from build123d import *

# Parameters (mm, degrees)
F4_R     = 2.9
F5_DEPTH = 75.0134427933
F6_SIZE  = 1.5
F7_COUNT = 3


with BuildPart() as f1:
    # F0 (on Front) → F1 (revolve)
    with BuildSketch(Plane.XZ):
        Polygon((-9.15, 1), (-9.15, 25), (-14, 25), (-25, 14.5), (-25, 10.5), (-14, 0), (-10.15, 0), (-10.15, 1), align=None)
    revolve(axis=Axis((0, 0, 12.5), (0, 0, -1)))

    # F2 (on Front) → F3 (revolve)
    with BuildSketch(Plane.XZ):
        Polygon((-35.94647469, -20.5244732297), (-15.2322022896, 1.1761930946), (-10.7806652787, 5.8397080583), (-15.0484629892, 9.9135149637), (-19.5, 5.25), (-40.2142724005, -16.4506663243), align=None)
    revolve(axis=Axis((-29.8571362002, 0, -5.6003331622), (0.6904757467, 0, 0.7233555441)))

    # F4 (on face) → F5 (cut, through all)
    with BuildSketch(Plane(origin=(-27.3888669951, 0, -28.6930987567), x_dir=(0.7233555441, 0, -0.6904757467), z_dir=(-0.6904757467, 0, -0.7233555441))):
        with Locations((-17.7304307809, 0)):
            Circle(F4_R)
    extrude(amount=-F5_DEPTH, mode=Mode.SUBTRACT)

    # F6
    f6_edges = [f1.edges().sort_by_distance(p)[0] for p in [
        (-44.48207, 0, -12.376859),
    ]]
    chamfer(f6_edges, length=F6_SIZE)

    # F7: F1 ×3 about axis
    f7_axis = Axis((0, 0, 14.5), (0, 0, -1))


with BuildPart() as f1_1:
    add(f1.part)
    for i in range(1, F7_COUNT):
        add(f1.part.rotate(f7_axis, i * 360 / F7_COUNT))


solid = f1_1.part
The model under review builds one solid part; all positions refer to its coordinate system, in mm. A direction names the side the tool comes from. Round coordinates to 2 decimals unless told otherwise and drop trailing zeros. Order: outer loops, then holes, each group sorted by start corner. A loop starts at its lowest first (then second) coordinate and runs counter-clockwise, first axis right, second up. Notation, with made-up numbers: (19.5, 55) -> (30.5, 55) arc R13 cw to (30.5, 70) -> close; hole circle Ø2 at (-2.5, 20.25). An arc over 180 degrees is marked (long way). Write item = value, one per line. Start each with the question number.
Item 1: For line 1 along Y through (x, z) = (0, 6.75); line 2 along X through (y, z) = (0, 16); line 3 along X through (y, z) = (0, 15.25), list the stretches that pass through material, from the lowest coordinate up.
Item 2: Clearance check with flat-ended pins moving along their axes: pin 1 Ø22.5 at (x, y) = (-1.5, 1) entering from -Z; pin 2 Ø10 at (x, z) = (11, 11) entering from +Y; pin 3 Ø4 at (x, z) = (12.5, 18) entering from -Y. State where each tip first meets the part, or that it passes through.
Item 3: Mouldability with a two-part tool opening along Z and no side actions: class faces 1 (the face through (16.53, -23.74, -6.78)), 2 (the face through (12.294, 26.184, -6.775)), 3 (the face through (20.246, -37.145, -14.468)), 4 (the face through (3, -9, 25)) as released by +Z, released by -Z, zero draft, split by the parting line, or undercut.
Item 4: Consider section B-B on y = 0. Write out the cut boundary in (x, z).
Item 5: For faces 5 (the face through (5, 8, 1)), 6 (the face through (-19.47, -0.04, 5.22)), 7 (the face through (17.2, 35.6, -17.2)), list the 3-axis set-ups (+Z, -Z, +X, -X, +Y, -Y) from which the entire face can be reached by the end or side of a thin tool; tool diameter is ignored.
Item 6: Consider section A-A on x = 0. Write out the cut boundary in (y, z).
Item 7: Consider section C-C on z = -10. Count the separate pieces of the cut face and the enclosed holes in it, plus the area to 3 significant figures.
Conclusion:
q1.line_1 = -21.07 to -9.15, 9.15 to 21.07
q1.line_2 = -23.43 to -9.15, 9.15 to 23.43
q1.line_3 = -24.21 to -9.15, 9.15 to 24.21
q2.pin_1 = 0
q2.pin_2 = 24.27
q2.pin_3 = -20.1
q3.face_1 = undercut
q3.face_2 = undercut
q3.face_3 = released by -Z
q3.face_4 = released by +Z
q4.outline = (-43.45, -11.29) -> (-43.4, -13.41) -> (-42.31, -14.45) -> (-21.6, 7.25) -> (-17.4, 3.25) -> (-38.12, -18.45) -> (-37.03, -19.49) -> (-34.91, -19.44) -> (-15.23, 1.18) -> (-14, 0) -> (-10.15, 0) -> (-10.15, 1) -> (-9.15, 1) -> (-9.15, 25) -> (-14, 25) -> (-25, 14.5) -> (-25, 10.5) -> (-23.77, 9.32) -> close; (9.15, 1) -> (10.15, 1) -> (10.15, 0) -> (14, 0) -> (25, 10.5) -> (25, 14.5) -> (14, 25) -> (9.15, 25) -> close
q5.face_5 = -Z
q5.face_6 = none
q5.face_7 = -Z, +X, +Y
q6.outline = (-25, 10.5) -> (-14, 0) -> (-10.15, 0) -> (-10.15, 1) -> (-9.15, 1) -> (-9.15, 25) -> (-14, 25) -> (-25, 14.5) -> close; (9.15, 1) -> (10.15, 1) -> (10.15, 0) -> (14, 0) -> (25, 10.5) -> (25, 14.5) -> (14, 25) -> (9.15, 25) -> close
q7.separate_pieces = 3
q7.enclosed_holes = 3
q7.area = 344 mm2
